Could you check a few things on this model? Use its own coordinates, in mm. A direction names the side the tool comes from. Give positions to 0.01 mm unless a question says otherwise; leave off trailing zeros. Order: outer loops, then holes, each group sorted by start corner. A loop starts at its lowest first (then second) coordinate and runs counter-clockwise, first axis right, second up. Notation, with made-up numbers: (1, 80.5) - (11, 80.5) arc R22 cw to (11, 87.5) - close; hole circle Ø3 at (-38.75, 55). An arc over 180 degrees is marked (long way). One line per question, with ' | ' between items. Start each with the question number.
1. Imagine slicing it at A-A (y = 10). Please give me the cut outline in (x, z).
2. Imagine slicing it at C-C (y = 30). Please give me the cut outline in (x, z).
3. If we mould it in two halves opening along Y, with no side actions, what happens to faces 4 (the flat face through (3, 0, 6)), 5 (the cylindrical face through (2.03, 10.07, 17.5)), 6 (the flat face through (6, 20, 2)), 7 (the flat face through (0, 20, 10))? For each: released by +Y, released by -Y, zero draft, split by the parting line, or undercut.
4. Imagine slicing it at B-B (z = 16). Please give me the cut outline in (x, y).
5. Which directions (+Z, -Z, +X, -X, +Y, -Y) give clear straight access to the entire face, cutting with the end or side of a thin tool? Please do faces 1 (the flat face through (2, 20, 21)), 2 (the cylindrical face through (1.3, 30.14, 2.99)), 3 (the flat face through (4, 20, 12)).
6. Imagine slicing it at D-D (x = 1.25). Please give me the cut outline in (y, z), and give its area (3 significant figures).
7. I need wall thicknesses on probe 1 along Y at (x, z) = (2.1, 16); probe 2 along X at (y, z) = (3, 20); probe 3 along X at (y, z) = (29, 2). Which ranges of each line are inside material? Lowest first, please. Write a range as from..to.
8. For P1, Ø12, axis at y = 13.5, z = 15, coming from the +X side; P2, Ø1, axis at y = 5, z = 10.5, coming from the -X side; P3, Ø1, axis at x = 3.5, y = 26, coming from the -Z side; P4, Ø12, axis at y = 27, z = 7.5, coming from the +X side, each with a flat end and sliding along its axis, tell me the tip position at first contact or that it passes through.
```python
from build123d import *

# Parameters (mm, degrees)
SKETCH1_W           = 4
SKETCH1_H           = 40
EXTRUDE_THIN2_DEPTH = 21
SKETCH4_R           = 4
SKETCH15_R          = 4.03
SKETCH15_R_2        = 2.2
CUT_EXTRUDE14_DEPTH = 20
SKETCH13_R          = 1.5
CUT_EXTRUDE10_DEPTH = 46.354161882


with BuildPart() as part:
    # Sketch1 → Extrude-Thin2 (new body)
    with BuildSketch(Plane.XY):
        with Locations((2, 20)):
            Rectangle(SKETCH1_W, SKETCH1_H)
    extrude(amount=EXTRUDE_THIN2_DEPTH)

    # Sweep3: sweep along a curve in space
    with BuildLine() as sweep3_path:
        Line((4, 0, 0), (4, 40, 0))
    # Sketch4 → Sweep3 (sweep)
    with BuildSketch(Plane(origin=(0, 40, 0), x_dir=(1, 0, 0), z_dir=(0, 1, 0))):
        with Locations((4, 0)):
            Circle(SKETCH4_R)
    sweep(path=sweep3_path.line)

    # Sketch15 → Cut-Extrude14 (cut)
    with BuildSketch(Plane(origin=(0, 40, 0), x_dir=(1, 0, 0), z_dir=(0, 1, 0))):
        with Locations((4, 0)):
            Circle(SKETCH15_R)
        with Locations(Location((4, 0, 0), (0, 0, 270))):
            Circle(SKETCH15_R_2, mode=Mode.SUBTRACT)
    extrude(amount=-CUT_EXTRUDE14_DEPTH, mode=Mode.SUBTRACT)

    # Sketch13 → Cut-Extrude10 (cut, through all)
    with BuildSketch(Plane(origin=(4, 0, 0), x_dir=(0, 0, -1), z_dir=(1, 0, 0))):
        with Locations((-16, 30)):
            Circle(SKETCH13_R)
        with Locations((-16, 10)):
            Circle(SKETCH13_R)
    extrude(amount=-CUT_EXTRUDE10_DEPTH, mode=Mode.SUBTRACT)


solid = part.part
```
Results found:
1) outline: (0, 0) arc R4 ccw (long way) to (4, 4) - (4, 14.5) - (0, 14.5) - close; (0, 17.5) - (4, 17.5) - (4, 21) - (0, 21) - close
2) outline: (0, 0.49) arc R4.03 cw to (4, 4.03) - (4, 14.5) - (0, 14.5) - close; (0, 17.5) - (4, 17.5) - (4, 21) - (0, 21) - close; circle Ø4.4 at (4, 0)
3) face 4: released by -Y | face 5: undercut | face 6: released by +Y | face 7: zero draft
4) outline: (0, 0) - (4, 0) - (4, 8.5) - (0, 8.5) - close; (0, 11.5) - (4, 11.5) - (4, 28.5) - (0, 28.5) - close; (0, 31.5) - (4, 31.5) - (4, 40) - (0, 40) - close
5) face 1: +Z, +X, -X, +Y, -Y | face 2: +Y | face 3: +Z, +X, +Y, -Y
6) outline: (0, -2.9) - (20, -2.9) - (20, 2.95) - (40, 2.95) - (40, 21) - (0, 21) - close; hole circle Ø3 at (10, 16); hole circle Ø3 at (30, 16) | area: 825 mm2
7) probe 1: y = 0..8.5, 11.5..28.5, 31.5..40 | probe 2: x = 0..4 | probe 3: x = 0..0.5, 3.08..4.92
8) P1: stops at x = 4 | P2: stops at x = 0 | P3: stops at z = -2.2 | P4: stops at x = 5.61
